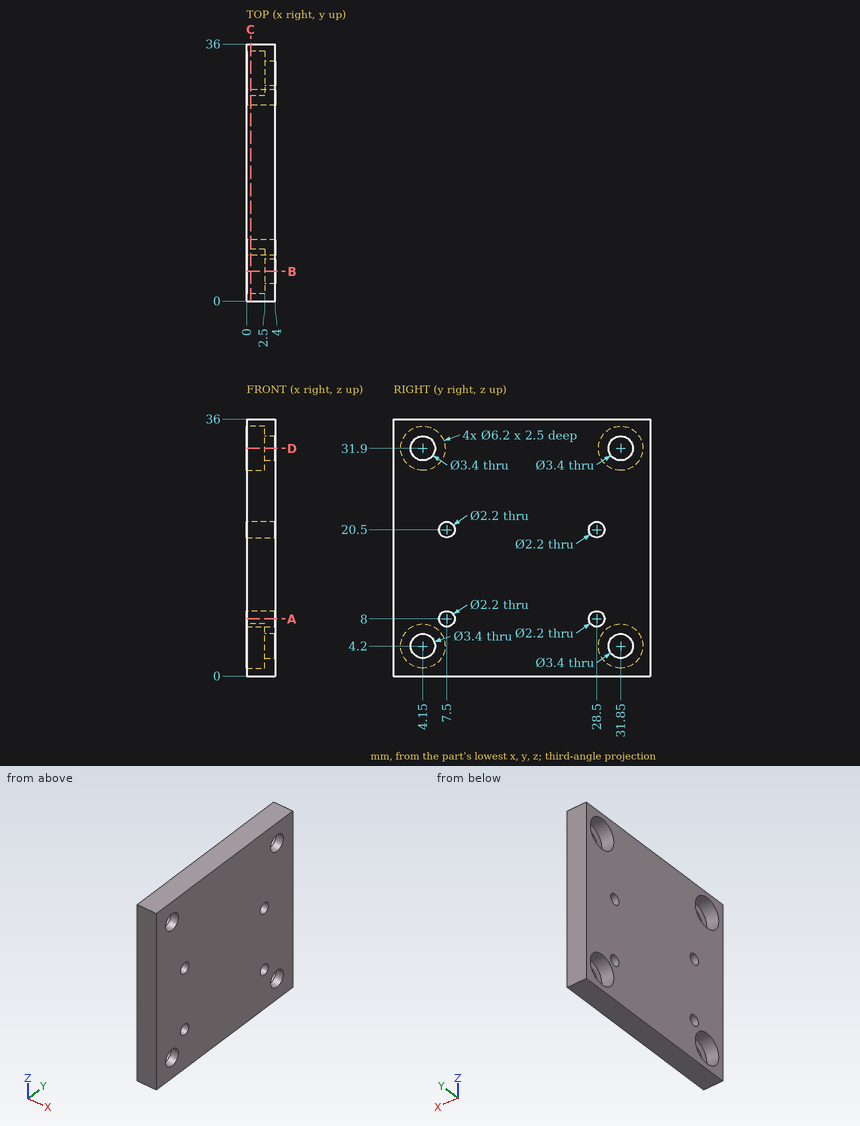
Here's the drawing with two shaded views (mm, measured from the low corner). I have some questions. Coordinates: 2 decimals unless noted, no trailing zeros. Write each loop counter-clockwise with the first axis right and the second up, starting at its lowest first coordinate (ties: lowest second). Pieces come first, ordered by that corner, then holes. Notation, with made-up numbers: M -11,40 L -5,40 A25 cw -5,54 Z; hole C 75,32 d4. An arc over 180 degrees is marked long. Write item = value, one per line. Start each with the question number.
Q1. If we section it at A-A, the plane z = 8: Write out the boundary of the cut face in (x, y), then the cut area to 3 significant figures.
Q2. I'm going to push flat-ended pins straight in: pin 1 (2 mm diameter, centred on y = 7.5, z = 20.5, fed in from +X); pin 2 (1.9 mm diameter, centred on y = 31, z = 30.5, fed in from -X). Where does each tip first touch, or does it pass through?
Q3. If we section it at C-C, the plane x = 0.55: State how many separate pieces and enclosed holes the cut face has, then the cut area to 3 significant figures.
Q4. If we section it at B-B, the plane y = 4.15: Write out the boundary of the cut face in (x, z), then the cut area to 3 significant figures.
Q5. If I drill on L1, parallel to Y at x = 1.55, z = 4.2; L2, parallel to Z at x = 3, y = 7.5; L3, parallel to Z at x = 0.95, y = 4, over which ranges is the centre line in solid material (lowest first)? Write a range as [from, to].
Q6. If we section it at D-D, the plane z = 31.9: Write out the boundary of the cut face in (x, y), then the cut area to 3 significant figures.
Check sheet entries:
q1.outline = M 0,0 L 4,0 L 4,6.4 L 0,6.4 Z; M 0,8.6 L 4,8.6 L 4,27.4 L 0,27.4 Z; M 0,29.6 L 4,29.6 L 4,36 L 0,36 Z
q1.area = 126 mm²
q2.pin_1 = through
q2.pin_2 = 2.5
q3.separate_pieces = 1
q3.enclosed_holes = 8
q3.area = 1,160 mm²
q4.outline = M 0,0 L 4,0 L 4,2.5 L 2.5,2.5 L 2.5,1.1 L 0,1.1 Z; M 0,7.3 L 2.5,7.3 L 2.5,5.9 L 4,5.9 L 4,30.2 L 2.5,30.2 L 2.5,28.8 L 0,28.8 Z; M 0,35 L 2.5,35 L 2.5,33.6 L 4,33.6 L 4,36 L 0,36 Z
q4.area = 103 mm²
q5.L1 = [0, 1.05], [7.25, 28.75], [34.95, 36]
q5.L2 = [0, 6.9], [9.1, 19.4], [21.6, 36]
q5.L3 = [0, 1.1], [7.3, 28.8], [35, 36]
q6.outline = M 0,0 L 4,0 L 4,2.45 L 2.5,2.45 L 2.5,1.05 L 0,1.05 Z; M 0,7.25 L 2.5,7.25 L 2.5,5.85 L 4,5.85 L 4,30.15 L 2.5,30.15 L 2.5,28.75 L 0,28.75 Z; M 0,34.95 L 2.5,34.95 L 2.5,33.55 L 4,33.55 L 4,36 L 0,36 Z
q6.area = 103 mm²
